```python
from build123d import *

# Parameters (mm, degrees)
EXTRUDE_1_DEPTH     = 25.5
M5X0_81_D           = 4.2
HOLE_WIZARD_6_0_1_D = 6
CHAMFER_1_SIZE      = 0.5


with BuildPart() as part:
    # Эскиз1 → Бобышка-Вытянуть1 (new body)
    with BuildSketch(Plane.XY):
        Polygon((110.285, 12.475), (110.285, 0), (0, 0), (0, 12.475), (9.956213203, 12.475), (11.65, 14.168786797), (13.343786797, 12.475), (27.356213203, 12.475), (29.05, 14.168786797), (30.743786797, 12.475), (44.756213203, 12.475), (46.45, 14.168786797), (48.143786797, 12.475), (62.156213203, 12.475), (63.85, 14.168786797), (65.543786797, 12.475), (79.556213203, 12.475), (81.25, 14.168786797), (82.943786797, 12.475), (96.956213203, 12.475), (98.65, 14.168786797), (100.343786797, 12.475), align=None)
    extrude(amount=-EXTRUDE_1_DEPTH)

    # Отверстие обработанное метчиком M5x0.81 (through all)
    with Locations(Plane(origin=(-77.729263736, 6.808390477, 0), x_dir=(1, 0, 0), z_dir=(0, 0, 1))):
        with Locations((132.879263736, -1.818390477), (87.879263736, -1.818390477), (177.879263736, -1.818390477)):
            Hole(M5X0_81_D / 2)

    # Отверстия под штифты Ø6.0 мм1 (through all)
    with Locations(Plane.XY):
        with Locations((32.65, 4.99), (77.65, 4.99)):
            Hole(HOLE_WIZARD_6_0_1_D / 2)

    # Фаска1
    chamfer_1_edges = [part.edges().sort_by_distance(p)[0] for p in [
        (0, 6.2375, 0),
        (55.1425, 0, 0),
        (110.285, 6.2375, 0),
        (0, 0, -12.75),
        (110.285, 0, -12.75),
        (55.1425, 0, -25.5),
    ]]
    chamfer(chamfer_1_edges, length=CHAMFER_1_SIZE)


solid = part.part
```
Geometry check sheet. Reference: the model listing, model coordinates, mm. A direction names the side the tool comes from. Give positions to 0.01 mm unless a question says otherwise; leave off trailing zeros. Order: outer loops, then holes, each group sorted by start corner. A loop starts at its lowest first (then second) coordinate and runs counter-clockwise, first axis right, second up.
1. Section check D-D, the plane x = 17. Enter the section's corners in (y, z) (3 decimals).
2. Thickness scan on L1, parallel to Y at x = 55.15, z = -6.25 (3 decimals); L2, parallel to X at y = 4.75, z = -22.5 (3 decimals); L3, parallel to X at y = 2.25, z = -8.25 (3 decimals). Record the ranges inside material, lowest first.
3. Gauge pin test, flat ends, axial feed: pin 1 Ø8 at (x, z) = (3, -17) entering from +Y (3 decimals); pin 2 Ø2 at (x, z) = (13, -6.5) entering from +Y; pin 3 Ø11 at (x, z) = (105, -14) entering from +Y; pin 4 Ø4 at (x, y) = (55.15, 4.99) entering from +Z. Record the tip position at first contact, or that the pin passes through.
4. Release check for a two-part mould opening along X. For faces 1 (the face through (110.285, 7, -13)), 2 (the face through (9.181, 3.127, -12.928)), 3 (the face through (56, 0, -13)) record: pulls with the +X half, pulls with the -X half, needs draft (parallel to the pull), parting line crosses it, or undercut.
5. Access from +Z, -Z, +X, -X, +Y, -Y to the whole of each face (thin tool, end or side, straight path). Record for faces 4 (the face through (38, 12.475, -13)), 5 (the face through (5, 12.475, -13)), 6 (the face through (0, 6, -13)), 7 (the face through (55.9, 7.4, 0)), 8 (the face through (105, 12.475, -13)).
6. Section check A-A, the plane y = 4.99. Enter the section's corners in (x, z) (3 decimals).
7. Section check C-C, the plane x = 32.65. Enter the section's corners in (y, z) (3 decimals).
8. Section check B-B, the plane z = -14.5. Give the number of separate pieces and of enclosed holes in the cut face, and give its area (3 significant figures).
Values follow:
1. outline: (0, -25) - (0.5, -25.5) - (12.475, -25.5) - (12.475, 0) - (0.5, 0) - (0, -0.5) - close
2. L1: y = 0 to 2.89, 7.09 to 12.475
2. L2: x = 0 to 8.064, 12.236 to 29.66, 35.64 to 53.064, 57.236 to 74.66, 80.64 to 98.064, 102.236 to 110.285
2. L3: x = 0 to 31.428, 33.872 to 76.428, 78.872 to 110.285
3. pin 1: stops at y = 12.475
3. pin 2: stops at y = 13.82
3. pin 3: stops at y = 13.32
3. pin 4: passes through
4. face 1: pulls with the +X half
4. face 2: undercut
4. face 3: needs draft
5. face 4: +Z, -Z, +Y
5. face 5: +Z, -Z, -X, +Y
5. face 6: +Z, -Z, -X, +Y, -Y
5. face 7: +Z, +X, -X, +Y, -Y
5. face 8: +Z, -Z, +X, +Y
6. outline: (0, -25.5) - (8.05, -25.5) - (8.05, 0) - (0.5, 0) - (0, -0.5) - close; (12.25, -25.5) - (29.65, -25.5) - (29.65, 0) - (12.25, 0) - close; (35.65, -25.5) - (53.05, -25.5) - (53.05, 0) - (35.65, 0) - close; (57.25, -25.5) - (74.65, -25.5) - (74.65, 0) - (57.25, 0) - close; (80.65, -25.5) - (98.05, -25.5) - (98.05, 0) - (80.65, 0) - close; (102.25, -25.5) - (110.285, -25.5) - (110.285, -0.5) - (109.785, 0) - (102.25, 0) - close
7. outline: (0, -25) - (0.5, -25.5) - (1.99, -25.5) - (1.99, 0) - (0.5, 0) - (0, -0.5) - close; (7.99, -25.5) - (12.475, -25.5) - (12.475, 0) - (7.99, 0) - close
8. separate pieces: 1
8. enclosed holes: 5
8. area: 1,290 mm2
